Study the drawing (mm; zero at the part's minimum x, y, z) and answer. Give positions to 0.01 mm unless a question says otherwise; leave off trailing zeros. Write each loop counter-clockwise with the first axis right and the second up, starting at its lowest first coordinate (ties: lowest second). Pieces come first, ordered by that corner, then holes.
1) Find section B-B (y = 39). Determine the outline of the cut face in (x, z).
2) Given pin 1 Ø1 at (x, z) = (200, 66.5) entering from -Y; pin 2 Ø8 at (x, z) = (179, 87) entering from +Y; pin 3 Ø3 at (x, y) = (83.5, 141) entering from -Z, each flat-ended and moving along its own axis, determine where each tip first touches the part or whether it passes through.
3) Straight lines are drawn through the part: probe 1 along Y at (x, z) = (112, 13); probe 2 along Y at (x, z) = (112.1, 85). For each, find the intervals that lie inside material, in ascending order.
4) Determine the mould class of the marked faces 1, 2, 3 and 4 for opening direction Y: pulls with the +Y half, pulls with the -Y half, needs draft (parallel to the pull), parting line crosses it, or undercut.
5) Find section A-A (x = 112.1). Determine the outline of the cut face in (y, z), plus the area to 3 significant figures.
6) Find section C-C (z = 117). Determine the outline of the cut face in (x, y), plus the area to 3 significant figures.
7) Find section D-D (z = 22.5). Determine the outline of the cut face in (x, y), plus the area to 3 significant figures.
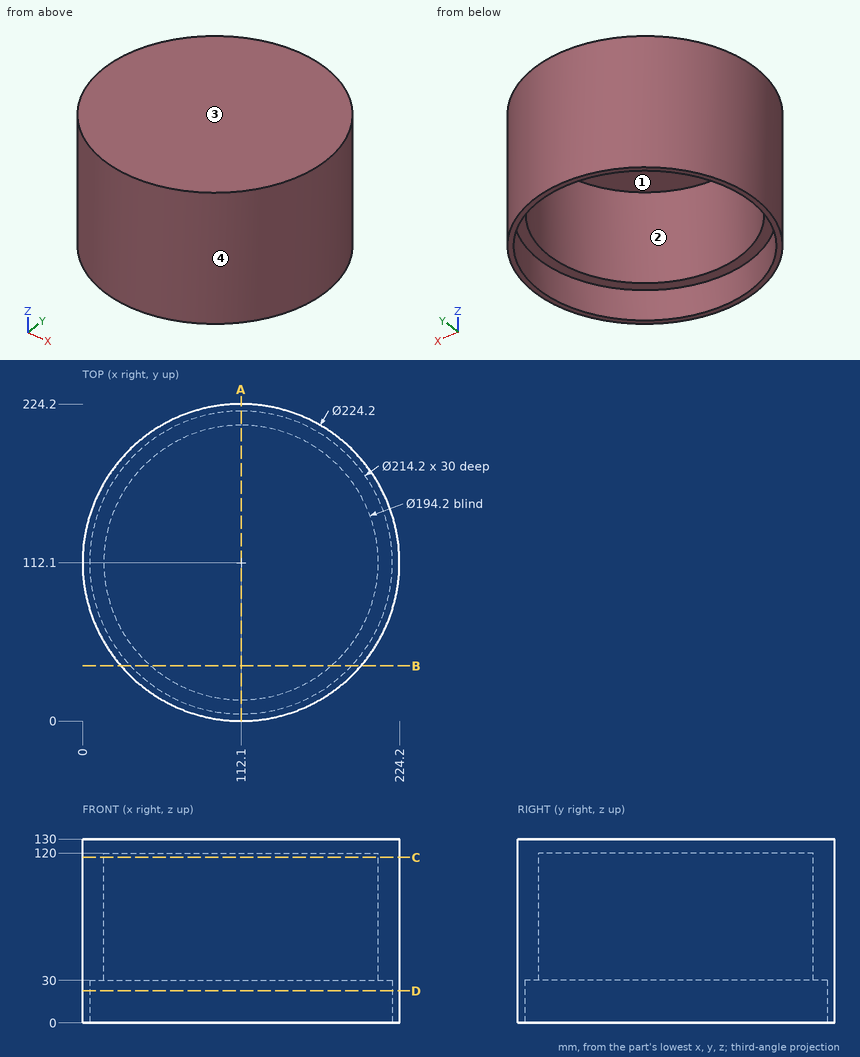
Results:
1. outline: (27.11, 0) - (33.83, 0) - (33.83, 30) - (48.19, 30) - (48.19, 120) - (176.01, 120) - (176.01, 30) - (190.37, 30) - (190.37, 0) - (197.09, 0) - (197.09, 130) - (27.11, 130) - close
2. pin 1: stops at y = 41.9
2. pin 2: stops at y = 204.89
2. pin 3: stops at z = 120
3. probe 1: y = 0 to 5, 219.2 to 224.2
3. probe 2: y = 0 to 15, 209.2 to 224.2
4. face 1: undercut
4. face 2: undercut
4. face 3: needs draft
4. face 4: parting line crosses it
5. outline: (0, 0) - (5, 0) - (5, 30) - (15, 30) - (15, 120) - (209.2, 120) - (209.2, 30) - (219.2, 30) - (219.2, 0) - (224.2, 0) - (224.2, 130) - (0, 130) - close
5. area: 5,240 mm2
6. outline: circle Ø224.2 at (112.1, 112.1); hole circle Ø194.2 at (112.1, 112.1)
6. area: 9,860 mm2
7. outline: circle Ø224.2 at (112.1, 112.1); hole circle Ø214.2 at (112.1, 112.1)
7. area: 3,440 mm2
